Geometry: see drawing. Coordinates: mm, zero at the bounding-box minimum. A direction names the side the tool comes from. Give positions to 0.01 mm unless a question says otherwise; leave off trailing zeros. Loops run counter-clockwise (first coordinate to the right, second up) from the corner with the lowest first, then second, coordinate; pieces in that order, holes last. Notation, with made-up numbers: (20.5, 83) -> (77.5, 83) arc R24 cw to (77.5, 115) -> close; hole circle Ø3 at (33, 32.25). An arc over 180 degrees is marked (long way). Return JSON: item names as keys, results as strings. Group by question number.
(1) Access query for the marked faces 4 and 5. Directions: +Z, -Z, +X, -X, +Y, -Y. A direction counts if a zero-diameter tool reaches every point of the face in a straight line with its end or side. Return the directions, or none.
(2) Ray query, line 1 (Z direction, x = 68.5, y = 40.5); line 2 (X direction, y = 45.5, z = 18.5); line 3 (X direction, y = 22, z = 5). Return the intervals inside material, ascending. Write a range as from..to.
(3) Cut plane A-A on x = 42. Return loops of the section in (y, z), then the cut area to 3 significant figures.
(4) Draft query along Z for the marked faces 1, 2 and 3. Return one class per face: released by +Z, released by -Z, zero draft, split by the parting line, or undercut.
(5) Cut plane D-D on x = 63. Return loops of the section in (y, z), then the cut area to 3 significant figures.
(6) Cut plane B-B on y = 19. Return loops of the section in (x, z), then the cut area to 3 significant figures.
(7) Pin query (flat end, axial travel): pin 1 (24 mm diameter, centred on y = 35.5, z = 29.5, fed in from +X); pin 2 (1.5 mm diameter, centred on x = 63, z = 11.5, fed in from -Y); pin 3 (10 mm diameter, centred on x = 44, z = 27.5, fed in from +Y). Return the tip coordinate at first contact, or that it passes through.
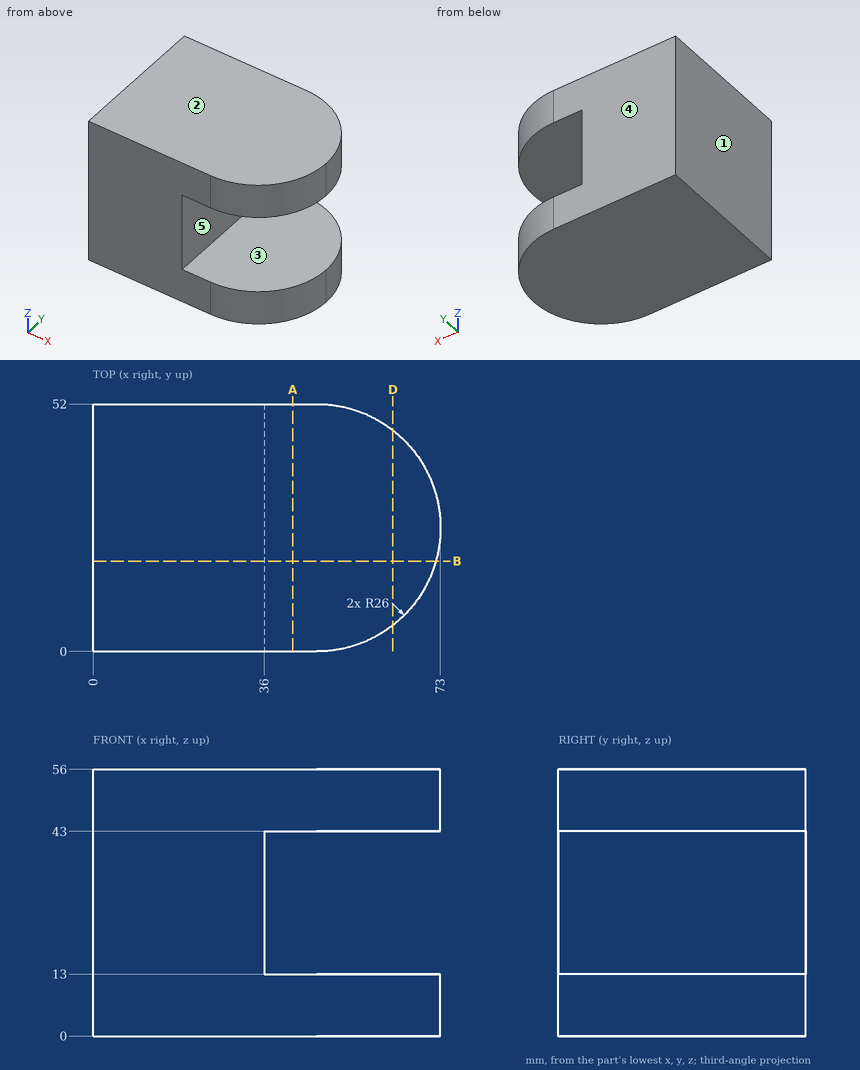
Answers:
{
 "1": {"face 4": "+Z, -Z, +X, -X, +Y", "face 5": "+X, +Y, -Y"},
 "2": {"line 1": "0..13, 43..56", "line 2": "0..36", "line 3": "0..72.69"},
 "3": {"outline": "(0, 0) -> (52, 0) -> (52, 13) -> (0, 13) -> close; (0, 43) -> (52, 43) -> (52, 56) -> (0, 56) -> close", "area": "1,350 mm²"},
 "4": {"face 1": "zero draft", "face 2": "released by +Z", "face 3": "undercut"},
 "5": {"outline": "(5.51, 0) -> (46.49, 0) -> (46.49, 13) -> (5.51, 13) -> close; (5.51, 43) -> (46.49, 43) -> (46.49, 56) -> (5.51, 56) -> close", "area": "1,070 mm²"},
 "6": {"outline": "(0, 0) -> (72.04, 0) -> (72.04, 13) -> (36, 13) -> (36, 43) -> (72.04, 43) -> (72.04, 56) -> (0, 56) -> close", "area": "2,950 mm²"},
 "7": {"pin 1": "x = 36", "pin 2": "y = 4.94", "pin 3": "through"}
}
